```python
from build123d import *

# Parameters (mm, degrees)
F0_W     = 127.497956
F0_H     = 61.302628
F0_W_2   = 111.95644
F0_H_2   = 48.063566
F1_DEPTH = 25.4
F3_D     = 6.35


with BuildPart() as f1:
    # F0 (on Top) → F1 (new body)
    with BuildSketch(Plane.XY):
        Rectangle(F0_W, F0_H)
        Rectangle(F0_W_2, F0_H_2, mode=Mode.SUBTRACT)
    extrude(amount=F1_DEPTH)

    # F3 (through all)
    with Locations(Plane.YZ.offset(63.748978)):
        with Locations((-24.319587, 6.187824), (-13.670773, 6.187824), (0, 6.187824), (12.231745, 6.187824), (23.743972, 6.187824)):
            Hole(F3_D / 2)


solid = f1.part
```
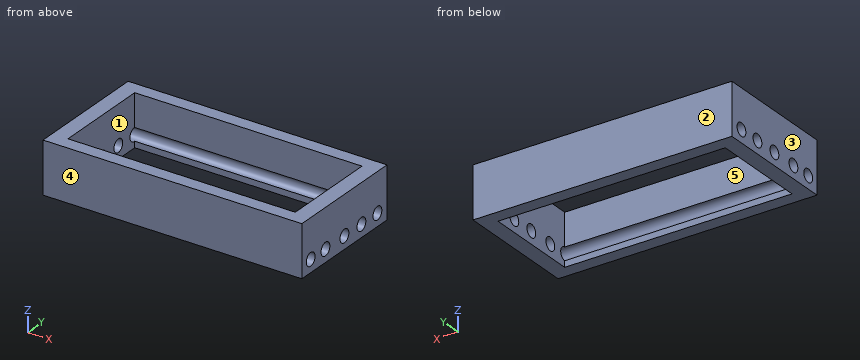
The model under review builds one solid part; all positions refer to its coordinate system, in mm. Face numbers are marked on the shaded views. A direction names the side the tool comes from. Give positions to 0.01 mm unless a question says otherwise; leave off trailing zeros. Write each loop counter-clockwise with the first axis right and the second up, starting at its lowest first coordinate (ties: lowest second). Pieces come first, ordered by that corner, then holes.
(1) Consider section B-B, the plane x = -20.5. Give the boundary of the cut face in (y, z) (3 decimals), and give its area (3 significant figures).
(2) Tool access review of the marked faces 1 and 2: name each direction out of +Z, -Z, +X, -X, +Y, -Y from which nothing blocks a thin tool from reaching the whole face with its end or side.
(3) To check wall thickness, follow L1, parallel to Y at x = 39, z = 11.75; L2, parallel to X at y = -18, z = 12.5; L3, parallel to Z at x = -60, y = 0. State the ranges of each line that lie inside material, in increasing order.
(4) Consider section A-A, the plane y = 0. Give the boundary of the cut face in (x, z).
(5) The part is to be moulded in two halves that separate along X. For the marked faces 3, 4 and 5, say which applies: released by +X, released by -X, zero draft, split by the parting line, or undercut.
(6) Consider section D-D, the plane z = 23.25. Give the boundary of the cut face in (x, y), and give its area (3 significant figures).
(7) Consider section C-C, the plane y = 7.5. Give the boundary of the cut face in (x, z).
Returned:
1. outline: (-30.651, 0) - (-24.032, 0) - (-24.032, 3.026) arc R3.175 cw (long way) to (-24.032, 9.35) - (-24.032, 25.4) - (-30.651, 25.4) - close; (24.032, 0) - (30.651, 0) - (30.651, 25.4) - (24.032, 25.4) - (24.032, 9.35) arc R3.175 cw to (24.032, 3.026) - close
1. area: 305 mm2
2. face 1: +Z, -Z
2. face 2: +Z, -Z, +X, -X, +Y
3. L1: y = -30.65 to -24.03, 24.03 to 30.65
3. L2: x = -63.75 to -55.98, 55.98 to 63.75
3. L3: z = 0 to 3.01, 9.36 to 25.4
4. outline: (-63.75, 0) - (-55.98, 0) - (-55.98, 3.01) - (-63.75, 3.01) - close; (-63.75, 9.36) - (-55.98, 9.36) - (-55.98, 25.4) - (-63.75, 25.4) - close; (55.98, 0) - (63.75, 0) - (63.75, 3.01) - (55.98, 3.01) - close; (55.98, 9.36) - (63.75, 9.36) - (63.75, 25.4) - (55.98, 25.4) - close
5. face 3: released by -X
5. face 4: zero draft
5. face 5: undercut
6. outline: (-63.75, -30.65) - (63.75, -30.65) - (63.75, 30.65) - (-63.75, 30.65) - close; hole (-55.98, -24.03) - (55.98, -24.03) - (55.98, 24.03) - (-55.98, 24.03) - close
6. area: 2,430 mm2
7. outline: (-63.75, 0) - (-55.98, 0) - (-55.98, 25.4) - (-63.75, 25.4) - close; (55.98, 0) - (63.75, 0) - (63.75, 25.4) - (55.98, 25.4) - close
